Read the model definition and answer for the solid it produces. Units are mm, in the model's axes. A direction names the side the tool comes from. Coordinates: 2 decimals unless noted, no trailing zeros. Write each loop counter-clockwise with the first axis right and the second up, starting at its lowest first coordinate (ties: lowest second). Pieces come first, ordered by that corner, then holes. Notation, with made-up numbers: (77, 72) - (108, 72) arc R37 cw to (108, 111) - close; hole circle Ø1 at (87.5, 59). An arc over 180 degrees is marked (long way). Return JSON: item names as keys, results as strings.
Autodesk Inventor part; units mm, degrees
ref_plane "YZ Plane" through (0, 0, 0) normal (1, 0, 0) x (0, 1, 0)
ref_plane "XZ Plane" through (0, 0, 0) normal (0, 1, 0) x (-1, 0, 0)
ref_plane "XY Plane" through (0, 0, 0) normal (0, 0, 1) x (1, 0, 0)
sketch "Sketch1" plane through (0, 0, 0) normal (0, 1, 0) x (-1, 0, 0)
  line L0 (0, 0) -> (84, 0)
  line L1 (84, 0) -> (84, -90)
  line L2 (84, -90) -> (0, -90)
  line L3 (0, -90) -> (0, 0)
  line L4 (84, 0) -> (76, 0)
  line L5 (76, 0) -> (4, 0)
  line L6 (4, 0) -> (4, -15.5)
  line L7 (4, -15.5) -> (76, -15.5)
  line L8 (76, -15.5) -> (76, 0)
  line L9 (84, -45) -> (0, -45) construction
  line L10 (4, -90) -> (4, -74.5)
  line L11 (4, -74.5) -> (76, -74.5)
  line L12 (76, -74.5) -> (76, -90)
  point P0 (4, 0)
  point P1 (4, -90)
  dimension "d0" = 84
  dimension "d1" = 90
  dimension "d4" = 8
  dimension "d5" = 72
  dimension "d6" = 15.5
extrude "Extrusion1" add sketch "Sketch1" along normal blind 4 contours L0 L6 L7 L8 L1 L2 L12 L11 L10 L3
sketch "Sketch2" plane through (0, 0, 0) normal (0, -1, 0) x (1, 0, 0)
  line L0 (-84, -90) -> (-84, 0)
  line L1 (-76, 0) -> (-76, -15.5)
  line L2 (-84, -90) -> (-76, -90)
  line L3 (-76, -90) -> (-76, 0)
  line L4 (-76, 0) -> (-84, 0)
  line L5 (-84, 0) -> (-84, -90)
  line L6 (0, -90) -> (0, 0)
  line L7 (0, 0) -> (0, -90)
  line L8 (-4, 0) -> (0, 0)
  line L9 (0, -90) -> (-4, -90)
  line L10 (-4, -90) -> (-4, 0)
  line L11 (-4, 0) -> (0, 0)
  line L12 (0, 0) -> (0, -90)
  dimension "d12" = 4
extrude "Extrusion2" add sketch "Sketch2" along normal blind 37
sketch "Sketch3" plane through (0, -37, 0) normal (0, -1, 0) x (1, 0, 0)
  line L0 (-76, -74.5) -> (-76, -90)
  line L1 (-76, -74.5) -> (-76, -73.5)
  line L2 (-76, -15.5) -> (-76, -74.5)
  line L3 (-76, -73.5) -> (-84, -73.5)
  line L4 (-84, -73.5) -> (-84, -16.5)
  line L5 (-84, -16.5) -> (-76, -16.5)
  line L6 (-76, -16.5) -> (-76, -73.5)
  point P0 (0, 0)
  dimension "d17" = 1
  dimension "d18" = 8
  dimension "d19" = 57
extrude "Extrusion3" add sketch "Sketch3" along normal blind 5
sketch "Sketch5" plane through (0, -37, 0) normal (0, -1, 0) x (1, 0, 0)
  line L0 (-4, -74.5) -> (-4, -73.5)
  line L1 (-4, -73.5) -> (-4, -73.5) construction
  line L2 (-4, 0) -> (-4, -90)
  line L3 (-4, -73.5) -> (0, -73.5)
  line L4 (0, -73.5) -> (0, -16.5)
  line L5 (0, -16.5) -> (-4, -16.5)
  line L6 (-4, -16.5) -> (-4, -73.5)
  point P0 (0, 0)
  dimension "d20" = 1
  dimension "d21" = 4
  dimension "d22" = 57
extrude "Extrusion4" add sketch "Sketch5" along normal blind 2
fillet "Fillet1" radius 2 6 edges at (-76, 2, -15.5) (-76, 0, -45) (-76, 2, -74.5) (-4, 2, -74.5) (-4, 0, -45) (-4, 2, -15.5)
sketch "Sketch6" plane through (0, 4, 0) normal (0, 1, 0) x (1, 0, 0)
  line L0 (-6, 74.5) -> (-74, 74.5)
  line L1 (-26.2554, 74.5) -> (0, 74.5) construction
  line L2 (0, 74.5) -> (-10, 74.5)
  line L3 (-10, 74.5) -> (-10, 72.5)
  line L4 (-10, 72.5) -> (0, 72.5)
  line L5 (0, 72.5) -> (0, 74.5)
  line L6 (-100.2554, 74.5) -> (-74, 74.5) construction
  line L7 (-84, 74.5) -> (-84, 72.5)
  line L8 (-84, 72.5) -> (-74, 72.5)
  line L9 (-74, 74.5) -> (-84, 74.5)
  line L10 (-74, 72.5) -> (-74, 74.5)
  line L11 (-26.2554, 17.5) -> (0, 17.5) construction
  line L12 (-10, 17.5) -> (-10, 15.5)
  line L13 (-10, 15.5) -> (0, 15.5)
  line L14 (0, 17.5) -> (-10, 17.5)
  line L15 (0, 15.5) -> (0, 17.5)
  line L16 (-100.2554, 17.5) -> (-74, 17.5) construction
  line L17 (-84, 17.5) -> (-84, 15.5)
  line L18 (-84, 15.5) -> (-74, 15.5)
  line L19 (-74, 17.5) -> (-84, 17.5)
  line L20 (-74, 15.5) -> (-74, 17.5)
  line L21 (-84, 0) -> (-76, 0)
  line L22 (-84, 0) -> (-76, 0)
  line L23 (-76, 0) -> (-76, 15.5)
  line L24 (-76, 15.5) -> (-84, 15.5)
  line L25 (-84, 15.5) -> (-84, 0)
  line L26 (-76, 76.5) -> (-76, 90)
  line L27 (-76, 90) -> (-84, 90)
  line L28 (-84, 90) -> (-84, 74.5)
  line L29 (-84, 74.5) -> (-76, 74.5)
  line L30 (-76, 74.5) -> (-76, 90)
  line L31 (-4, 90) -> (-4, 76.5)
  line L32 (-4, 90) -> (0, 90)
  line L33 (0, 90) -> (0, 74.5)
  line L34 (0, 74.5) -> (-4, 74.5)
  line L35 (-4, 74.5) -> (-4, 90)
  line L36 (-4, 0) -> (0, 0)
  line L37 (-4, 0) -> (0, 0)
  line L38 (0, 0) -> (0, 15.5)
  line L39 (0, 15.5) -> (-4, 15.5)
  line L40 (-4, 15.5) -> (-4, 0)
  dimension "d26" = 10
  dimension "d27" = 2
  dimension "d30" = 74
  dimension "d33" = 57
extrude "Extrusion5" add sketch "Sketch6" along normal blind 9
fillet "Fillet2" radius 2 4 edges at (-76, 8.5, -15.5) (-4, 8.5, -15.5) (-4, 8.5, -74.5) (-76, 8.5, -74.5)
sketch "Sketch8" plane through (-84, -42, -73.5) normal (-1, 0, 0) x (0, 0, 1)
  line L0 (-16.5, 5) -> (-16.5, 55)
  line L1 (-16.5, 5) -> (8, 5)
  line L2 (0, 3) -> (57, 3)
  line L3 (-16.5, 5) -> (8, 5) construction
  line L4 (24, 5) -> (24, 20)
  line L5 (24, 20) -> (8, 20)
  line L6 (8, 20) -> (8, 5)
  line L7 (57, 0) -> (0, 0)
  line L8 (8, 5) -> (8, 0)
  line L9 (8, 0) -> (24, 0)
  line L10 (24, 0) -> (24, 5)
  line L11 (73.5, 5) -> (73.5, 55)
  line L12 (73.5, 5) -> (54, 5)
  line L13 (54, 5) -> (54, 20)
  line L14 (54, 20) -> (73.5, 20)
  line L15 (73.5, 20) -> (73.5, 5)
  line L16 (54, 20) -> (41, 20)
  line L17 (41, 20) -> (41, 0)
  line L18 (41, 0) -> (54, 0)
  line L19 (54, 0) -> (54, 20)
  point P0 (73.5, 42)
  dimension "d39" = 24.5
  dimension "d40" = 0
  dimension "d41" = 16
  dimension "d42" = 15
  dimension "d44" = 19.5
  dimension "d45" = 15
  dimension "d46" = 13
extrude "Extrusion6" cut sketch "Sketch8" against normal up to surface (8 mm away) contours L8 L6 L5 L4 L10 L2 | L2 L10 L7 L8 | L17 L16 L13 L19 L2 | L2 L19 L7 L17
properties part number "Breadboard_insert"
(1) A cutting plane is placed at A-A (z = -84). Determine the outline of the cut face in (x, y).
Answer:
{"outline": "(-84, -37) - (-76, -37) - (-76, 13) - (-84, 13) - close; (-4, -37) - (0, -37) - (0, 13) - (-4, 13) - close"}
(2) Straight lines are drawn through the part: line 1 (X direction, y = -13, z = -20); line 2 (Y direction, x = -66, z = -72.5); line 3 (X direction, y = -28, z = -29.5). For each, find the intervals that lie inside material, in ascending order. Write a range as from..to.
Answer:
{"line 1": "-84..-76, -4..0", "line 2": "0..4", "line 3": "-4..0"}
(3) A cutting plane is placed at B-B (y = -31.5). Determine the outline of the cut face in (x, z), and give its area (3 significant figures).
Answer:
{"outline": "(-84, -90) - (-76, -90) - (-76, -65.5) - (-84, -65.5) - close; (-84, -49.5) - (-76, -49.5) - (-76, -32.5) - (-84, -32.5) - close; (-84, -19.5) - (-76, -19.5) - (-76, 0) - (-84, 0) - close; (-4, -90) - (0, -90) - (0, 0) - (-4, 0) - close", "area": "848 mm²"}
(4) Which of the six approach directions +Z, -Z, +X, -X, +Y, -Y give full straight-line access (tool end or side, diameter ignored) to faces 1 (the face through (-80, -32, -32.5)), 2 (the face through (-2, -39, -45)), 3 (the face through (-80, -37, -82)), 4 (the face through (-2, -37, -8))?
Answer:
{"face 1": "-X, -Y", "face 2": "+Z, -Z, +X, -Y", "face 3": "-Z, +X, -X, -Y", "face 4": "+Z, +X, -X, -Y"}
(5) A cutting plane is placed at C-C (y = -12). Determine the outline of the cut face in (x, z).
Answer:
{"outline": "(-84, -90) - (-76, -90) - (-76, 0) - (-84, 0) - close; (-4, -90) - (0, -90) - (0, 0) - (-4, 0) - close"}
(6) Determine the mould class of faces 5 (the face through (-2, -12, -90)), 6 (the face through (-76, -15, -46)), 7 (the face through (-79, 8, -72.5)) for opening direction Z: +Z half, -Z half, draft (parallel to the pull), parting line (faces both ways), or undercut.
Answer:
{"face 5": "-Z half", "face 6": "draft", "face 7": "undercut"}
(7) A cutting plane is placed at D-D (y = 2). Determine the outline of the cut face in (x, z), and give its area (3 significant figures).
Answer:
{"outline": "(-84, -90) - (-76, -90) - (-76, -76.5) arc R2 cw to (-74, -74.5) - (-6, -74.5) arc R2 cw to (-4, -76.5) - (-4, -90) - (0, -90) - (0, 0) - (-4, 0) - (-4, -13.5) arc R2 cw to (-6, -15.5) - (-74, -15.5) arc R2 cw to (-76, -13.5) - (-76, 0) - (-84, 0) - close", "area": "5,330 mm²"}
(8) Flat-ended cylindrical pins translate along their axes: P1, Ø1.2, axis at x = -1.5, z = -83, coming from the -Y side; P2, Ø0.6, axis at x = -1, y = -38.5, coming from the +Z side; P3, Ø6.5, axis at x = -80.5, z = -57.5, coming from the -Y side; P4, Ø1, axis at x = -5.5, z = -76, coming from the +Y side. Find the tip coordinate at first contact, or state that the pin passes through.
Answer:
{"P1": "y = -37", "P2": "z = -16.5", "P3": "y = -22", "P4": "through"}
